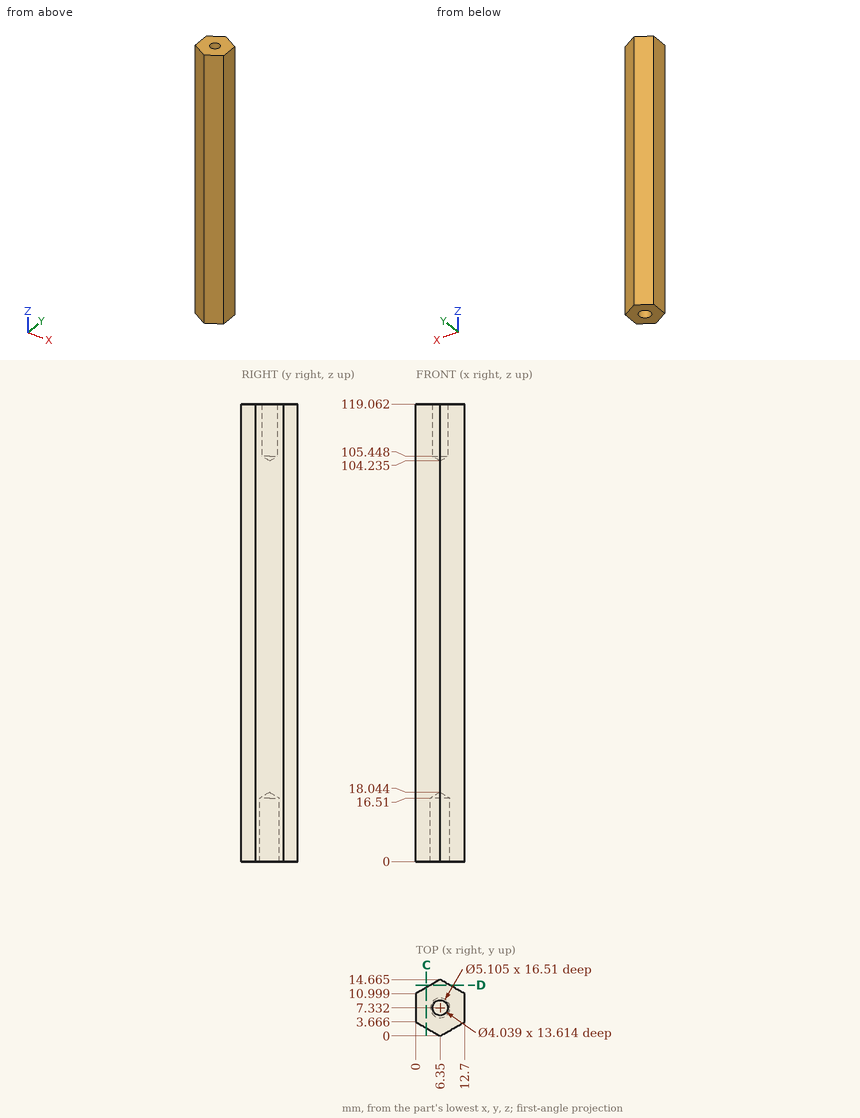
Part print with two shaded views. Sizes in mm from the minimum x, y, z corner. Round coordinates to 2 decimals unless told otherwise and drop trailing zeros. Write each loop counter-clockwise with the first axis right and the second up, starting at its lowest first coordinate (ties: lowest second). Pieces come first, ordered by that corner, then holes. Notation, with made-up numbers: M 10,-17 L 37,-17 A23 cw 37,2 Z; hole C 75,80.25 d1. An arc over 180 degrees is marked long. Use CSV: the item, a comma, the result in double quotes.
1. Saw through at D-D (y = 13.25). Give the cut face in (x, z).
Reply:
outline,"M 3.9,0 L 8.8,0 L 8.8,119.06 L 3.9,119.06 Z"
2. Wall check: probe 1 along Y at (x, z) = (6.35, 6.75) (1 decimal); probe 2 along Z at (x, y) = (8, 9.25) (1 decimal); probe 3 along X at (y, z) = (14.25, 59) (1 decimal). Give the ranges that are in metal, low to high. Write a range as from..to.
Reply:
probe 1,"y = 0..4.8, 9.9..14.7"
probe 2,"z = 16.5..119.1"
probe 3,"x = 5.6..7.1"
3. Saw through at C-C (x = 2.75). Give the cut face in (y, z), plus the area to 3 significant figures.
Reply:
outline,"M 2.08,0 L 12.59,0 L 12.59,119.06 L 2.08,119.06 Z"
area,"1,250 mm²"
4. Flat gauge pins, fed straight in: pin 1 (4.5 mm diameter, centred on x = 6.35, y = 7.33, fed in from -Z); pin 2 (5 mm diameter, centred on x = 3, z = 44.5, fed in from +Y) (1 decimal). Where does each tip first touch, or does it go through?
Reply:
pin 1,"stops at z = 16.69"
pin 2,"stops at y = 14.2"
